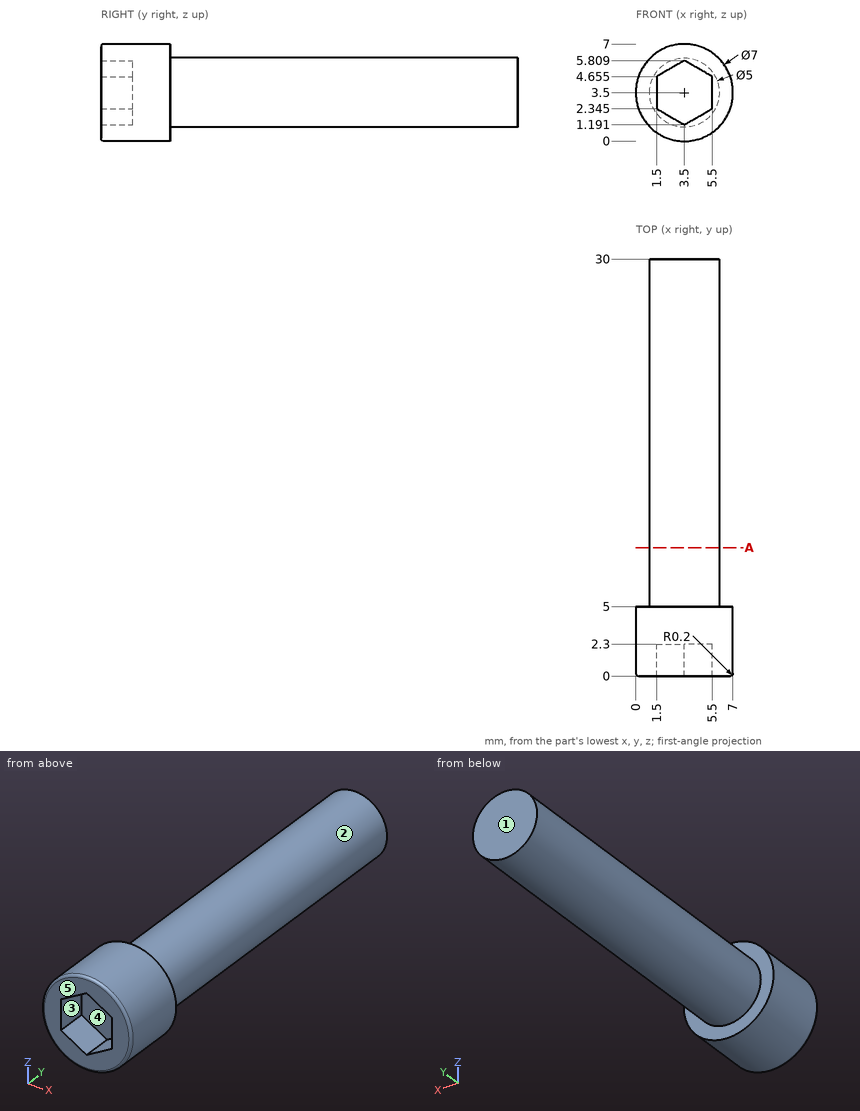
The figure shows three views and two pictorial views of one solid part (mm, origin at its lowest corner). Answer the questions. A direction names the side the tool comes from. Coordinates: 2 decimals unless noted, no trailing zeros. Loops run counter-clockwise (first coordinate to the right, second up) from the corner with the lowest first, then second, coordinate; pieces in that order, holes last. Notation, with made-up numbers: (45, 26.25) -> (86, 26.25) arc R15 cw to (86, 42.25) -> close; hole circle Ø1 at (-26.5, 79.5). An arc over 180 degrees is marked (long way). Write item = value, one per line. Start each with the question number.
1) A cutting plane is placed at A-A (y = 9.25). Give the vertices of the cut face in (x, z), then the cut area to 3 significant figures.
2) Given pin 1 Ø0.7 at (y, z) = (0.5, 3) entering from +X; pin 2 Ø1 at (x, y) = (3.5, 20) entering from -Z; pin 3 Ø2 at (x, z) = (4, 4.5) entering from -Y; pin 4 Ø4 at (y, z) = (11.5, 4) entering from +X, each flat-ended and moving along its own axis, determine where each tip first touches the part or whether it passes through.
3) Straight lines are drawn through the part: line 1 (Z direction, x = 5, y = 15.75); line 2 (Y direction, x = 4.5, z = 3.25); line 3 (Y direction, x = 1.5, z = 5.5). For each, find the intervals that lie inside material, in ascending order. Write a range as from..to.
4) The mould has two halves that part along X. Classify the marked faces 1, 2 and 3: released by +X, released by -X, zero draft, split by the parting line, or undercut.
5) A tool of negligible diameter and unlimited length cuts with its end or side. For the marked faces 4 and 5, from which of +Z, -Z, +X, -X, +Y, -Y can it reach the whole face along a straight path? Write none if from no direction.
Responses:
q1.outline = circle Ø5 at (3.5, 3.5)
q1.area = 19.6 mm²
q2.pin_1 = 7
q2.pin_2 = 1
q2.pin_3 = 0
q2.pin_4 = 6
q3.line_1 = 1.5..5.5
q3.line_2 = 2.3..30
q3.line_3 = 0..5
q4.face_1 = zero draft
q4.face_2 = split by the parting line
q4.face_3 = undercut
q5.face_4 = -Y
q5.face_5 = +Z, -Z, +X, -X, -Y
